from build123d import *
from OCP.BRepFilletAPI import BRepFilletAPI_MakeChamfer

# Parameters (mm, degrees)
EXTRUDE_1_DEPTH = 50
CHAMFER_1_SIZE  = 5
CHAMFER_1_SIZE2 = 3.535533906
CHAMFER_2_SIZE  = 1


with BuildPart() as part:
    # 草图1 → 凸台-拉伸1 (new body)
    with BuildSketch(Plane(origin=(0, 0, 0), x_dir=(1, 0, 0), z_dir=(0, 1, 0))):
        Polygon((0, 0), (50, 50), (50, 0), align=None)
    extrude(amount=EXTRUDE_1_DEPTH)

    # 倒角1: one chamfer whose edges measure the first distance from different faces: ONE call of the kernel's chamfer builder (chamfer() names one face for all edges)
    chamfer_1_edges_1 = [part.edges().sort_by_distance(p)[0] for p in [
        (0, 25, 0),
    ]]
    chamfer_1_side_1 = [part.faces().sort_by_distance(p)[0] for p in [
        (25, 25, -25),
    ]]
    chamfer_1_edges_2 = [part.edges().sort_by_distance(p)[0] for p in [
        (50, 25, -50),
    ]]
    chamfer_1_side_2 = [part.faces().sort_by_distance(p)[0] for p in [
        (50, 25, -25),
    ]]
    chamfer_1 = BRepFilletAPI_MakeChamfer(part.part.solid().wrapped)
    for e in chamfer_1_edges_1:
        chamfer_1.Add(CHAMFER_1_SIZE, CHAMFER_1_SIZE2, e.wrapped, chamfer_1_side_1[0].wrapped)  # the first distance lies on this face
    for e in chamfer_1_edges_2:
        chamfer_1.Add(CHAMFER_1_SIZE, CHAMFER_1_SIZE2, e.wrapped, chamfer_1_side_2[0].wrapped)  # the first distance lies on this face
    add(Compound.cast(chamfer_1.Shape()), mode=Mode.REPLACE)

    # 倒角2
    chamfer_2_edges = [part.edges().sort_by_distance(p)[0] for p in [
        (25.517766953, 0, -25.517766953),
        (25.517766953, 50, -25.517766953),
        (26.767766953, 0, 0),
        (3.535533906, 0, -1.767766953),
        (48.75, 0, -46.25),
        (26.767766953, 50, 0),
        (3.535533906, 50, -1.767766953),
        (48.75, 50, -46.25),
        (3.535533906, 25, 0),
        (50, 0, -22.5),
        (50, 25, 0),
        (50, 50, -22.5),
    ]]
    chamfer(chamfer_2_edges, length=CHAMFER_2_SIZE)


solid = part.part
For this review, take the finished solid that the model builds, in its own axes (mm). Round coordinates to 2 decimals unless told otherwise and drop trailing zeros. Loops run counter-clockwise (first coordinate to the right, second up) from the corner with the lowest first, then second, coordinate; pieces in that order, holes last. Notation, with made-up numbers: (-38, -26) - (-27, -26) arc R7 ccw to (-27, -18) - close; hole circle Ø6 at (78, -25). An arc over 180 degrees is marked (long way). One line per item, written item: value. Start each with the question number.
Item 1: Take a section at A-A (y = 39.5). Give the boundary of the cut face in (x, z), plus the area to 3 significant figures.
Item 2: Take a section at B-B (z = -31). Give the boundary of the cut face in (x, y).
Item 3: For L1, parallel to Z at x = 44, y = 16; L2, parallel to Z at x = 9, y = 30; L3, parallel to X at y = 3.5, z = -44, list the stretches that pass through material, from the lowest coordinate up.
Item 4: Take a section at C-C (x = 25). Give the boundary of the cut face in (y, z).
Item 5: Clearance check with flat-ended pins moving along their axes: pin 1 Ø3 at (x, y) = (11, 42) entering from -Z; pin 2 Ø1.5 at (x, z) = (18, -20.5) entering from -Y. State where each tip first meets the part, or that it passes through.
Answer below:
1. outline: (3.54, -3.54) - (47.5, -47.5) - (50, -45) - (50, -1) - (49, 0) - (4.54, 0) - (3.54, -1) - close
1. area: 1,240 mm2
2. outline: (31, 1) - (32.41, 0) - (49, 0) - (50, 1) - (50, 49) - (49, 50) - (32.41, 50) - (31, 49) - close
3. L1: z = -44 to 0
3. L2: z = -9 to 0
3. L3: x = 44 to 50
4. outline: (0, -23.59) - (1, -25) - (49, -25) - (50, -23.59) - (50, -1) - (49, 0) - (1, 0) - (0, -1) - close
5. pin 1: stops at z = -12.5
5. pin 2: passes through
